```python
from build123d import *

# Parameters (mm, degrees)
SKETCH1_W                                    = 60
SKETCH1_H                                    = 40
BOSS_EXTRUDE1_DEPTH                          = 11
SKETCH3_W                                    = 15
SKETCH3_H                                    = 6
SKETCH3_W_2                                  = 9.5
SKETCH3_H_2                                  = 2
CUT_EXTRUDE10_DEPTH                          = 61
CSK_FOR_M3_HEX_SOCKET_COUNTERSUNK_CA_2_COUNT = 2
CSK_FOR_M3_HEX_SOCKET_COUNTERSUNK_CA_2_PITCH = 25.167603026
CSK_FOR_M3_HEX_SOCKET_COUNTERSUNK_CA_3_COUNT = 2
CSK_FOR_M3_HEX_SOCKET_COUNTERSUNK_CA_3_PITCH = 40.419124333
CSK_FOR_M3_HEX_SOCKET_COUNTERSUNK_CA_4_COUNT = 2
CSK_FOR_M3_HEX_SOCKET_COUNTERSUNK_CA_4_PITCH = 31.627478082
SKETCH1_6_R                                  = 10
CUT_EXTRUDE19_DEPTH                          = 9
CUT_EXTRUDE21_START                          = 11
SKETCH1_7_R                                  = 3
CUT_EXTRUDE21_DEPTH                          = 12
SKETCH8_R                                    = 3.75
CUT_EXTRUDE22_DEPTH                          = 2
FILLET1_R                                    = 10


with BuildPart() as part:
    # Sketch1 → Boss-Extrude1 (new body)
    with BuildSketch(Plane(origin=(0, 0, 0), x_dir=(1, 0, 0), z_dir=(0, 1, 0))):
        Rectangle(SKETCH1_W, SKETCH1_H)
    extrude(amount=BOSS_EXTRUDE1_DEPTH)

    # Sketch3 → Cut-Extrude10 (cut, through all)
    with BuildSketch(Plane.ZY.offset(30)):
        with Locations((10.5, 6)):
            Rectangle(SKETCH3_W, SKETCH3_H)
        with Locations((-10.5, 6)):
            Rectangle(SKETCH3_W, SKETCH3_H)
        with Locations((-10.5, 10)):
            Rectangle(SKETCH3_W_2, SKETCH3_H_2)
        with Locations((10.5, 10)):
            Rectangle(SKETCH3_W_2, SKETCH3_H_2)
    extrude(amount=-CUT_EXTRUDE10_DEPTH, mode=Mode.SUBTRACT)

    # Sketch7 → CSK for M3 Hex Socket Countersunk Cap Screw2 (revolve, cut)
    with BuildSketch(Plane(origin=(15.813739041, 3, -12.583801513), x_dir=(0, 0, 1), z_dir=(1, 0, 0))):
        Polygon((0, 0), (0, 3), (1.75, 3), (1.75, 2), (3.75, 0), align=None)
    csk_for_m3_hex_socket_countersunk_cap_sc = revolve(axis=Axis((15.813739041, 9.35, -12.583801513), (0, -1, 0)), mode=Mode.SUBTRACT)

    # CSK for M3 Hex Socket Countersunk Ca 2: CSK for M3 Hex Socket Countersunk Cap Screw2 ×2
    with Locations(*[(0, 0, i * CSK_FOR_M3_HEX_SOCKET_COUNTERSUNK_CA_2_PITCH) for i in range(1, CSK_FOR_M3_HEX_SOCKET_COUNTERSUNK_CA_2_COUNT)]):
        add(csk_for_m3_hex_socket_countersunk_cap_sc, mode=Mode.SUBTRACT)

    # CSK for M3 Hex Socket Countersunk Ca 3: CSK for M3 Hex Socket Countersunk Cap Screw2 ×2
    with Locations(*[Vector(-0.782487958, 0, 0.622665717) * (i * CSK_FOR_M3_HEX_SOCKET_COUNTERSUNK_CA_3_PITCH) for i in range(1, CSK_FOR_M3_HEX_SOCKET_COUNTERSUNK_CA_3_COUNT)]):
        add(csk_for_m3_hex_socket_countersunk_cap_sc, mode=Mode.SUBTRACT)

    # CSK for M3 Hex Socket Countersunk Ca 4: CSK for M3 Hex Socket Countersunk Cap Screw2 ×2
    with Locations(*[(-i * CSK_FOR_M3_HEX_SOCKET_COUNTERSUNK_CA_4_PITCH, 0, 0) for i in range(1, CSK_FOR_M3_HEX_SOCKET_COUNTERSUNK_CA_4_COUNT)]):
        add(csk_for_m3_hex_socket_countersunk_cap_sc, mode=Mode.SUBTRACT)

    # Sketch1<6> → Cut-Extrude19 (cut)
    with BuildSketch(Plane(origin=(0, 0, 0), x_dir=(1, 0, 0), z_dir=(0, 1, 0))):
        Circle(SKETCH1_6_R)
    extrude(amount=CUT_EXTRUDE19_DEPTH, mode=Mode.SUBTRACT)

    # Sketch1<7> → Cut-Extrude21 (cut, through all)
    with BuildSketch(Plane(origin=(0, 0, 0), x_dir=(1, 0, 0), z_dir=(0, 1, 0)).offset(CUT_EXTRUDE21_START)):
        Circle(SKETCH1_7_R)
    extrude(amount=-CUT_EXTRUDE21_DEPTH, mode=Mode.SUBTRACT)

    # Sketch8 → Cut-Extrude22 (cut)
    with BuildSketch(Plane(origin=(0, 11, 0), x_dir=(1, 0, 0), z_dir=(0, 1, 0))):
        with Locations((-15.813739041, -12.583801513)):
            Circle(SKETCH8_R)
        with Locations((15.813739041, -12.583801513)):
            Circle(SKETCH8_R)
        with Locations((15.813739041, 12.583801513)):
            Circle(SKETCH8_R)
        with Locations((-15.813739041, 12.583801513)):
            Circle(SKETCH8_R)
    extrude(amount=-CUT_EXTRUDE22_DEPTH, mode=Mode.SUBTRACT)

    # Fillet1
    fillet1_edges = [part.edges().sort_by_distance(p)[0] for p in [
        (30, 5.5, -20),
        (30, 5.5, 20),
        (-30, 5.5, 20),
        (-30, 5.5, -20),
    ]]
    fillet(fillet1_edges, radius=FILLET1_R)


solid = part.part
```
For this review, take the finished solid that the model builds, in its own axes (mm). A direction names the side the tool comes from. Coordinates: 2 decimals unless noted, no trailing zeros. Write each loop counter-clockwise with the first axis right and the second up, starting at its lowest first coordinate (ties: lowest second). Pieces come first, ordered by that corner, then holes. Notation, with made-up numbers: (-4, 42.25) - (0, 42.25) arc R18 ccw to (0, 48.25) - close; hole circle Ø5 at (65, 11.5). An arc over 180 degrees is marked (long way). Answer in a Markdown table with one row per item. Add a question column.
Q1. For P1, Ø5, axis at y = 8, z = 13, coming from the -X side; P2, Ø1.8, axis at x = 23.5, y = 7, coming from the -Z side; P3, Ø1, axis at x = -22.5, y = 9.5, coming from the +Z side; P4, Ø3, axis at x = -15.81, z = -12.58, coming from the +Y side, all flat-tipped, find the tip position at first contact; note any pin that passes through.
Q2. We need section B-B, the plane z = 0. State the section outline as (x, y) points.
Q3. Draft analysis for pull direction X (two halves, no side actions). For faces 4 (the cylindrical face through (-3, 10, 0)), 5 (the flat face through (-30, 4, 0)), 6 (the cylindrical face through (-10, 2, 0)), 7 (the flat face through (0, 10, -5.75)), state which applies: +X half, -X half, draft (parallel to the pull), parting line (faces both ways), or undercut.
Q4. We need section C-C, the plane x = 8. State the section outline as (y, z) points.
Q5. We need section A-A, the plane y = 7. State the section outline as (x, z) points.
Q6. Tool access review of faces 1 (the flat face through (-24, 10, -15.25)), 2 (the flat face through (0, 6, 18)), 3 (the cylindrical face through (15.773, 10.014, 16.334)): name each direction out of +Z, -Z, +X, -X, +Y, -Y from which nothing blocks a thin tool from reaching the whole face with its end or side.
Q7. For probe 1 along Z at (x, y) = (-3, 7.5); probe 2 along Z at (x, y) = (-6.5, 10.5); probe 3 along X at (y, z) = (1.75, 11), list the stretches that pass through material, from the lowest coordinate up.
Q8. We need section D-D, the plane x = 0. State the section outline as (y, z) points, and give its area (3 significant figures).
Answer list:
| question | item | result |
|---|---|---|
| 1 | P1 | stops at x = -28.51 |
| 1 | P2 | stops at z = -19.66 |
| 1 | P3 | stops at z = 19.8 |
| 1 | P4 | passes through |
| 2 | outline | (-30, 0) - (-10, 0) - (-10, 9) - (-3, 9) - (-3, 11) - (-30, 11) - close; (3, 9) - (10, 9) - (10, 0) - (30, 0) - (30, 11) - (3, 11) - close |
| 3 | face 4 | undercut |
| 3 | face 5 | -X half |
| 3 | face 6 | undercut |
| 3 | face 7 | draft |
| 4 | outline | (0, -20) - (11, -20) - (11, -15.25) - (9, -15.25) - (9, -18) - (3, -18) - (3, -6) - (0, -6) - close; (0, 6) - (3, 6) - (3, 18) - (9, 18) - (9, 15.25) - (11, 15.25) - (11, 20) - (0, 20) - close; (9, -5.75) - (11, -5.75) - (11, 5.75) - (9, 5.75) - close |
| 5 | outline | (-30, -3) - (-9.54, -3) arc R10 cw to (-9.54, 3) - (-30, 3) - close; (-26, -18) arc R10 ccw to (-20, -20) - (20, -20) arc R10 ccw to (26, -18) - close; (-26, 18) - (26, 18) arc R10 ccw to (20, 20) - (-20, 20) arc R10 ccw to start; (9.54, -3) - (30, -3) - (30, 3) - (9.54, 3) arc R10 cw to start |
| 6 | face 1 | +X, -X, +Y |
| 6 | face 2 | +X, -X |
| 6 | face 3 | +Y |
| 7 | probe 1 | z = -20 to -18, 18 to 20 |
| 7 | probe 2 | z = -20 to -15.25, -5.75 to 5.75, 15.25 to 20 |
| 7 | probe 3 | x = -29.95 to -17.75, -13.88 to 13.88, 17.75 to 29.95 |
| 8 | outline | (0, -20) - (11, -20) - (11, -15.25) - (9, -15.25) - (9, -18) - (3, -18) - (3, -10) - (0, -10) - close; (0, 10) - (3, 10) - (3, 18) - (9, 18) - (9, 15.25) - (11, 15.25) - (11, 20) - (0, 20) - close; (9, -5.75) - (11, -5.75) - (11, -3) - (9, -3) - close; (9, 3) - (11, 3) - (11, 5.75) - (9, 5.75) - close |
| 8 | area | 114 mm2 |
